```python
from build123d import *


with BuildPart() as f2:
    # F2: sweep along a path in F1
    with BuildLine(Plane.XY) as f2_path:
        Line((-241.3, 0), (-241.3, 99.9497326006))
        Line((-241.3, 99.9497326006), (-99.9497326006, 241.3))
        Line((-99.9497326006, 241.3), (99.9497326006, 241.3))
        Line((99.9497326006, 241.3), (241.3, 99.9497326006))
        Line((241.3, 99.9497326006), (241.3, -99.9497326006))
        Line((241.3, -99.9497326006), (99.9497326006, -241.3))
        Line((99.9497326006, -241.3), (-99.9497326006, -241.3))
        Line((-99.9497326006, -241.3), (-241.3, -99.9497326006))
        Line((-241.3, -99.9497326006), (-241.3, 0))
    # F0 (on Front) → F2 (sweep)
    with BuildSketch(Plane.XZ):
        Polygon((-238.125, 38.1), (-241.3, 38.1), (-241.3, 0), (-203.2, 0), (-203.2, 3.175), (-238.125, 3.175), align=None)
    sweep(path=f2_path.line, transition=Transition.RIGHT)


solid = f2.part
```
Work out the finished part from the listing and answer in its coordinate system (mm). A direction names the side the tool comes from. Coordinates: 2 decimals unless noted, no trailing zeros. Order: outer loops, then holes, each group sorted by start corner. A loop starts at its lowest first (then second) coordinate and runs counter-clockwise, first axis right, second up. Notation, with made-up numbers: (-21, 40.25) - (22, 40.25) arc R29 cw to (22, 77.25) - close; hole circle Ø6 at (18.5, 82.25). An arc over 180 degrees is marked (long way). Answer as a JSON object with one key per item and string values.
1. Find section C-C on z = 14. Determine the outline of the cut face in (x, y) (3 decimals).
Output values:
{"outline": "(-241.3, -99.95) - (-99.95, -241.3) - (99.95, -241.3) - (241.3, -99.95) - (241.3, 99.95) - (99.95, 241.3) - (-99.95, 241.3) - (-241.3, 99.95) - close; hole (-238.125, -98.635) - (-98.635, -238.125) - (98.635, -238.125) - (238.125, -98.635) - (238.125, 98.635) - (98.635, 238.125) - (-98.635, 238.125) - (-238.125, 98.635) - close"}
2. The mould has two halves that part along X. Classify faces 4 (the face through (-142.85, 144.52, 1.57)), 5 (the face through (171.61, 169.64, 19.32)), 6 (the face through (-1, -241.3, 19)): +X half, -X half, draft (parallel to the pull), parting line (faces both ways), or undercut.
Output values:
{"face 4": "undercut", "face 5": "+X half", "face 6": "draft"}
3. Consider line 1 (X direction, y = 73, z = 18) (3 decimals); line 2 (Z direction, x = -142, y = 193) (3 decimals). Determine where each line is inside the solid, lowest interval first.
Output values:
{"line 1": "x = -241.3 to -238.125, 238.125 to 241.3", "line 2": "z = 0 to 3.175"}
4. Find section A-A on y = 77. Determine the outline of the cut face in (x, z) (3 decimals), plus the area to 3 significant figures.
Output values:
{"outline": "(-241.3, 0) - (-203.2, 0) - (-203.2, 3.175) - (-238.125, 3.175) - (-238.125, 38.1) - (-241.3, 38.1) - close; (203.2, 0) - (241.3, 0) - (241.3, 38.1) - (238.125, 38.1) - (238.125, 3.175) - (203.2, 3.175) - close", "area": "464 mm²"}
5. A tool of negligible diameter and unlimited length cuts with its end or side. For faces 1 (the face through (-167.4, 169.36, 20.39)), 2 (the face through (0, 204, 0)), 3 (the face through (144.52, 142.85, 1.57)), from which of +Z, -Z, +X, -X, +Y, -Y can it reach the whole face along a straight path? Write none if from no direction.
Output values:
{"face 1": "+Z", "face 2": "-Z, +X, -X, +Y, -Y", "face 3": "+Z, -Z"}
6. Each of these flat-tipped pins is pushed along its axis until it touches: P1, Ø12, axis at y = 125, z = 24, coming from the +X side; P2, Ø5, axis at x = -110, z = 32, coming from the +Y side; P3, Ø5, axis at y = -100.5, z = 14.5, coming from the +X side; P4, Ø3, axis at y = 173.5, z = 10.5, coming from the +X side. Where does it stop, or does it pass through?
Output values:
{"P1": "stops at x = 222.25", "P2": "stops at y = 233.75", "P3": "stops at x = 241.3", "P4": "stops at x = 169.25"}
